Design review of the part shown in the three views and the two pictorial views. Dimensions are in mm from the part's minimum x, y and z. A direction names the side the tool comes from. Give positions to 0.01 mm unless a question says otherwise; leave off trailing zeros. Loops run counter-clockwise (first coordinate to the right, second up) from the corner with the lowest first, then second, coordinate; pieces in that order, holes last. Notation, with made-up numbers: (-1.75, 44) -> (41.25, 44) arc R28 ccw to (41.25, 63) -> close; hole circle Ø7 at (13.25, -21.5). An arc over 180 degrees is marked (long way). Use CSV: the item, a comma, the result in double quotes. Start each with the question number.
Item 1: We need section C-C (x = 25). State the section outline as (y, z) points.
Item 2: Clearance check with flat-ended pins moving along their axes: pin 1 (4.5 mm diameter, centred on x = 18, z = 9.5, fed in from -Y); pin 2 (8 mm diameter, centred on x = 21.5, z = 14.5, fed in from +Y); pin 3 (13 mm diameter, centred on x = 35.5, y = 16, fed in from +Z). State where each tip first meets the part, or that it passes through.
Item 3: We need section B-B (z = 12.75). State the section outline as (x, y) points, plus the area to 3 significant figures.
Item 4: We need section D-D (x = 43). State the section outline as (y, z) points.
Item 5: We need section A-A (y = 65). State the section outline as (x, z) points, plus the area to 3 significant figures.
Item 6: The part is to be moulded in two halves that separate along Y. For the marked faces 1, 2 and 3, say which applies: +Y half, -Y half, draft (parallel to the pull), parting line (faces both ways), or undercut.
Item 7: Wall thickness on line 1 along Y through (x, z) = (21.5, 10.5); line 2 along Z through (x, y) = (41.5, 80.5); line 3 along Z through (x, y) = (24, 104): over which ranges is each line inside the solid? List them lowest first. Write a range as from..to.
Item 8: For the marked faces 4, 5 and 6, list the 3-axis set-ups (+Z, -Z, +X, -X, +Y, -Y) from which the entire face can be reached by the end or side of a thin tool; tool diameter is ignored.
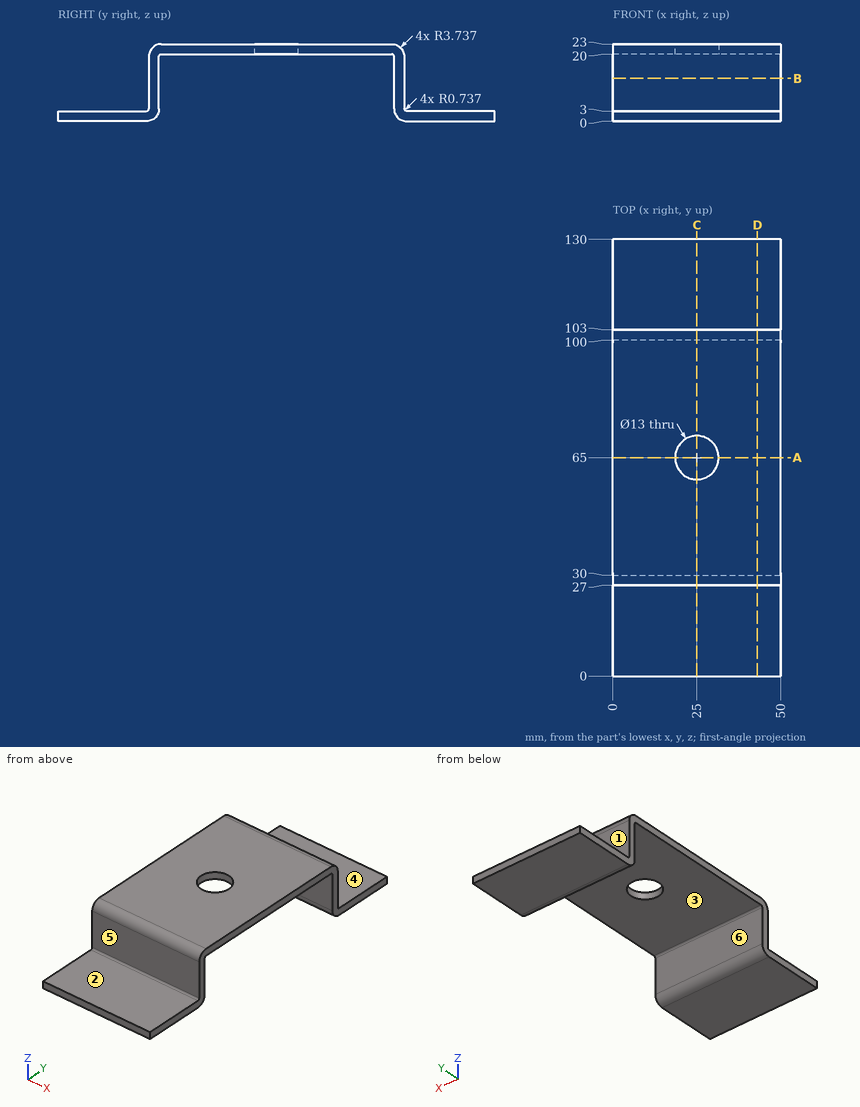
Results found:
1,outline,"(0, 0) -> (26.26, 0) arc R3.74 ccw to (30, 3.74) -> (30, 19.26) arc R0.74 cw to (30.74, 20) -> (58.5, 20) -> (58.5, 23) -> (30.74, 23) arc R3.74 ccw to (27, 19.26) -> (27, 3.74) arc R0.74 cw to (26.26, 3) -> (0, 3) -> close; (71.5, 20) -> (99.26, 20) arc R0.74 cw to (100, 19.26) -> (100, 3.74) arc R3.74 ccw to (103.74, 0) -> (130, 0) -> (130, 3) -> (103.74, 3) arc R0.74 cw to (103, 3.74) -> (103, 19.26) arc R3.74 ccw to (99.26, 23) -> (71.5, 23) -> close"
2,pin 1,"y = 27"
2,pin 2,"y = 103"
2,pin 3,"z = 3"
3,outline,"(0, 27) -> (50, 27) -> (50, 30) -> (0, 30) -> close; (0, 100) -> (50, 100) -> (50, 103) -> (0, 103) -> close"
3,area,"300 mm²"
4,outline,"(0, 0) -> (26.26, 0) arc R3.74 ccw to (30, 3.74) -> (30, 19.26) arc R0.74 cw to (30.74, 20) -> (99.26, 20) arc R0.74 cw to (100, 19.26) -> (100, 3.74) arc R3.74 ccw to (103.74, 0) -> (130, 0) -> (130, 3) -> (103.74, 3) arc R0.74 cw to (103, 3.74) -> (103, 19.26) arc R3.74 ccw to (99.26, 23) -> (30.74, 23) arc R3.74 ccw to (27, 19.26) -> (27, 3.74) arc R0.74 cw to (26.26, 3) -> (0, 3) -> close"
5,outline,"(0, 20) -> (18.5, 20) -> (18.5, 23) -> (0, 23) -> close; (31.5, 20) -> (50, 20) -> (50, 23) -> (31.5, 23) -> close"
5,area,"111 mm²"
6,face 1,"+Y half"
6,face 2,"draft"
6,face 3,"undercut"
7,line 1,"27..30, 100..103"
7,line 2,"20..23"
7,line 3,"0..3"
8,face 4,"+Z, +X, -X, +Y"
8,face 5,"+Z, +X, -X, -Y"
8,face 6,"-Z, +X, -X"
